from build123d import *

# Parameters (mm, degrees)
SKETCH1_R           = 10
BOSS_EXTRUDE1_DEPTH = 20
SKETCH2_R           = 24.856075314
SKETCH2_R_2         = 20
CUT_EXTRUDE3_DEPTH  = 20
SKETCH5_W           = 3
SKETCH5_H           = 20
CUT_EXTRUDE4_DEPTH  = 10
CUT_EXTRUDE5_START  = -20
SKETCH6_R           = 2.5
CUT_EXTRUDE5_DEPTH  = 25
SKETCH7_W           = 7
SKETCH7_H           = 8
CUT_EXTRUDE7_DEPTH  = 10
SKETCH8_R           = 0.5
CUT_EXTRUDE8_DEPTH  = 30
SKETCH9_W           = 2
SKETCH9_H           = 7.475145823
CUT_EXTRUDE9_DEPTH  = 23
SKETCH10_W          = 3
SKETCH10_H          = 24.206915905
CUT_EXTRUDE10_DEPTH = 2.5
SKETCH12_W          = 4
SKETCH12_H          = 4
CUT_EXTRUDE12_DEPTH = 15
BOSS_EXTRUDE7_DEPTH = 4
SKETCH39_R          = 2.5
CUT_EXTRUDE15_DEPTH = 12.5
BOSS_EXTRUDE8_DEPTH = 12.5
SKETCH42_R          = 0.6
CUT_EXTRUDE16_DEPTH = 33.5


with BuildPart() as part:
    # Sketch1 → Boss-Extrude1 (new body, symmetric)
    with BuildSketch(Plane(origin=(0, 0, 0), x_dir=(1, 0, 0), z_dir=(0, 1, 0))):
        Circle(SKETCH1_R)
    extrude(amount=BOSS_EXTRUDE1_DEPTH, both=True)

    # Sketch2 → Cut-Extrude3 (cut, symmetric)
    with BuildSketch(Plane.XY):
        Circle(SKETCH2_R)
        Circle(SKETCH2_R_2, mode=Mode.SUBTRACT)
    cut_extrude3 = extrude(amount=CUT_EXTRUDE3_DEPTH, both=True, mode=Mode.SUBTRACT)

    # Sketch5 → Cut-Extrude4 (cut)
    with BuildSketch(Plane(origin=(0, 20, 0), x_dir=(1, 0, 0), z_dir=(0, 1, 0))):
        Rectangle(SKETCH5_W, SKETCH5_H)
    cut_extrude4 = extrude(amount=-CUT_EXTRUDE4_DEPTH, mode=Mode.SUBTRACT)

    # Sketch6 → Cut-Extrude5 (cut)
    with BuildSketch(Plane.ZY.offset(-1.5).offset(CUT_EXTRUDE5_START)):
        with Locations((0, 13.943670675)):
            Circle(SKETCH6_R)
    cut_extrude5 = extrude(amount=CUT_EXTRUDE5_DEPTH, mode=Mode.SUBTRACT)

    # Sketch7 → Cut-Extrude7 (cut)
    with BuildSketch(Plane(origin=(0, 20, 0), x_dir=(1, 0, 0), z_dir=(0, 1, 0))):
        with Locations((5, 0)):
            Rectangle(SKETCH7_W, SKETCH7_H)
    cut_extrude7 = extrude(amount=-CUT_EXTRUDE7_DEPTH, mode=Mode.SUBTRACT)

    # Sketch8 → Cut-Extrude8 (cut)
    with BuildSketch(Plane(origin=(0, 10, 0), x_dir=(1, 0, 0), z_dir=(0, 1, 0))):
        with Locations((8, -3.414911062)):
            Circle(SKETCH8_R)
    cut_extrude8 = extrude(amount=-CUT_EXTRUDE8_DEPTH, mode=Mode.SUBTRACT)

    # Sketch9 → Cut-Extrude9 (cut)
    with BuildSketch(Plane(origin=(0, 10, 0), x_dir=(1, 0, 0), z_dir=(0, 1, 0))):
        with Locations((1.5, 7.737572912)):
            Rectangle(SKETCH9_W, SKETCH9_H)
    cut_extrude9 = extrude(amount=CUT_EXTRUDE9_DEPTH, mode=Mode.SUBTRACT)

    # Mirror2: Cut-Extrude3, Cut-Extrude4, Cut-Extrude5, Cut-Extrude7, Cut-Extrude8, Cut-Extrude9 across plane
    add(cut_extrude3.mirror(Plane.ZX), mode=Mode.SUBTRACT)
    add(cut_extrude4.mirror(Plane.ZX), mode=Mode.SUBTRACT)
    add(cut_extrude5.mirror(Plane.ZX), mode=Mode.SUBTRACT)
    add(cut_extrude7.mirror(Plane.ZX), mode=Mode.SUBTRACT)
    add(cut_extrude8.mirror(Plane.ZX), mode=Mode.SUBTRACT)
    add(cut_extrude9.mirror(Plane.ZX), mode=Mode.SUBTRACT)

    # Mirror3: Cut-Extrude8 across plane
    add(cut_extrude8.mirror(Plane.XY), mode=Mode.SUBTRACT)

    # Sketch10 → Cut-Extrude10 (cut)
    with BuildSketch(Plane(origin=(0, 10, 0), x_dir=(1, 0, 0), z_dir=(0, 1, 0))):
        with Locations((0, 0.041148578)):
            Rectangle(SKETCH10_W, SKETCH10_H)
    cut_extrude10 = extrude(amount=-CUT_EXTRUDE10_DEPTH, mode=Mode.SUBTRACT)

    # Mirror4: Cut-Extrude10 across plane
    add(cut_extrude10.mirror(Plane.ZX), mode=Mode.SUBTRACT)

    # Sketch12 → Cut-Extrude12 (cut, symmetric)
    with BuildSketch(Plane.XY):
        with Locations((-8, 0)):
            Rectangle(SKETCH12_W, SKETCH12_H)
        with Locations((8, 0)):
            Rectangle(SKETCH12_W, SKETCH12_H)
    extrude(amount=CUT_EXTRUDE12_DEPTH, both=True, mode=Mode.SUBTRACT)

    # Sketch37 → Boss-Extrude7 (add)
    with BuildSketch(Plane(origin=(0, 12.5, 0), x_dir=(1, 0, 0), z_dir=(0, 1, 0))):
        with BuildLine():
            Line((-2.5, 9.682458366), (-2.5, 12.247448714))
            ThreePointArc((-2.5, 12.247448714), (-7.90569415, -9.682458366), (12.5, 0))
            ThreePointArc((12.5, 0), (9.682458366, 7.90569415), (2.5, 12.247448714))
            Line((2.5, 12.247448714), (2.5, 9.682458366))
            ThreePointArc((2.5, 9.682458366), (7.90569415, 6.123724357), (10, 0))
            ThreePointArc((10, 0), (-6.123724357, -7.90569415), (-2.5, 9.682458366))
        make_face()
    boss_extrude7 = extrude(amount=-BOSS_EXTRUDE7_DEPTH)

    # Mirror5: Boss-Extrude7 across plane
    add(boss_extrude7.mirror(Plane.ZX))

    # Sketch39 → Cut-Extrude15 (cut)
    with BuildSketch(Plane(origin=(0, 0, 0), x_dir=(0, 0, -1), z_dir=(1, 0, 0))):
        with Locations((0, 13.943670675)):
            Circle(SKETCH39_R)
        with Locations((0, -13.943670675)):
            Circle(SKETCH39_R)
    extrude(amount=CUT_EXTRUDE15_DEPTH, mode=Mode.SUBTRACT)

    # Sketch41 → Boss-Extrude8 (add)
    with BuildSketch(Plane(origin=(0, 7.5, 0), x_dir=(1, 0, 0), z_dir=(0, 1, 0))):
        with BuildLine():
            Line((1.5, -6.25), (-1.5, -6.25))
            Line((-1.5, -6.25), (-1.5, -9.886859967))
            ThreePointArc((-1.5, -9.886859967), (0, -10), (1.5, -9.886859967))
            Line((1.5, -9.886859967), (1.5, -6.25))
        make_face()
    boss_extrude8 = extrude(amount=BOSS_EXTRUDE8_DEPTH)

    # Mirror6: Boss-Extrude8 across plane
    add(boss_extrude8.mirror(Plane.ZX))

    # Sketch42 → Cut-Extrude16 (cut, through all)
    with BuildSketch(Plane(origin=(0, 12.5, 0), x_dir=(1, 0, 0), z_dir=(0, 1, 0))):
        with Locations((11.25, 0)):
            Circle(SKETCH42_R)
    cut_extrude16 = extrude(amount=-CUT_EXTRUDE16_DEPTH, mode=Mode.SUBTRACT)

    # Mirror7: Cut-Extrude16 across plane
    add(cut_extrude16.mirror(Plane(origin=(0, 0, 0), x_dir=(0, 0, 1), z_dir=(1, 0, 0))), mode=Mode.SUBTRACT)


solid = part.part
Here's how the part is built. I have some questions about the finished solid (model axes, mm). A direction names the side the tool comes from. Round coordinates to 2 decimals unless told otherwise and drop trailing zeros. Loops run counter-clockwise (first coordinate to the right, second up) from the corner with the lowest first, then second, coordinate; pieces in that order, holes last. Notation, with made-up numbers: M 51.25,24.25 L 56.25,24.25 A30 cw 56.25,53.25 Z; hole C 81.5,-19 d9. An arc over 180 degrees is marked long. Write each question's results on one line, items separated by ' | '. Start each with the question number.
(1) I want a section at C-C (y = -9). Please give me the cut outline in (x, z), then the cut area to 3 significant figures.
(2) On a 3-axis mill with a long thin cutter (end or side, diameter ignored), from which of +Z, -Z, +X, -X, +Y, -Y can I reach the whole of each face in a straight line? I mean faces 1 (the cylindrical face through (10.084, 11.503, -0.542)), 2 (the flat face through (0.9, 8.5, 10.2)), 3 (the flat face through (0, -7.5, -2)), 4 (the flat face through (-8, 2, 0)). Say none if no direction works.
(3) I want a section at B-B (x = 0). Please give me the cut outline in (y, z).
(4) Thinking about a two-plate mould opening in X: for faces 5 (the cylindrical face through (-4.878, 19.396, -0.138)), 6 (the flat face through (5, -15, -4)), 7 (the flat face through (-7.5, 12.5, 7.4)), 8 (the cylindrical face through (8.74, 17.99, -0.03)), which applies, pulls with the +X half, pulls with the -X half, needs draft (parallel to the pull), parting line crosses it, or undercut?
(5) If I drill on probe 1 along Z at (x, y) = (8, 7.75); probe 2 along Y at (x, z) = (10.75, -4); probe 3 along X at (y, z) = (-9.5, -3.25), over which ranges is the centre line in solid material (lowest first)? Write a range as from..to.
(6) Will these pins go through, and if not, where does the flat tip stop? P1, Ø4, axis at x = 0.5, y = -1.5, coming from the +Z side; P2, Ø5, axis at y = -13, z = -0.5, coming from the +X side; P3, Ø8, axis at y = 13, z = 4.5, coming from the -X side; P4, Ø8, axis at x = -0.5, z = -9.5, coming from the +Y side.
(7) I want a section at D-D (x = -9). Please give me the cut outline in (y, z).
(8) I want a section at A-A (x = 9). Please give me the cut outline in (y, z), then the cut area to 3 significant figures.
Solved:
1) outline: M -2.5,-12.25 L -2.5,-9.68 A10 ccw -1.5,-9.89 L -1.5,6.25 L 1.5,6.25 L 1.5,-9.89 A10 ccw 2.5,-9.68 L 2.5,-12.25 A12.5 ccw long Z; hole C -11.25,0 d1.2; hole C 8,-3.41 d1; hole C 8,3.41 d1; hole C 11.25,0 d1.2 | area: 426 mm²
2) face 1: +X | face 2: none | face 3: -Z, -Y | face 4: +Z, -Z, -X
3) outline: M -20,6.25 L -7.5,6.25 L -7.5,-10 L 7.5,-10 L 7.5,6.25 L 20,6.25 L 20,10 L 12.5,10 L 12.5,12.5 L 8.5,12.5 L 8.5,10 L -8.5,10 L -8.5,12.5 L -12.5,12.5 L -12.5,10 L -20,10 Z
4) face 5: pulls with the -X half | face 6: undercut | face 7: needs draft | face 8: pulls with the +X half
5) probe 1: z = -6..-3.91, -2.91..2.91, 3.91..6 | probe 2: y = -12.5..-8.5, 8.5..12.5 | probe 3: x = -12.07..-1.5, 1.5..7.53, 8.47..12.07
6) P1: stops at z = 10 | P2: stops at x = 12.5 | P3: stops at x = -12.49 | P4: stops at y = 19.94
7) outline: M -17.86,-4.36 L -12.5,-4.36 L -12.5,-8.67 L -8.5,-8.67 L -8.5,-4.36 L -2,-4.36 L -2,4.36 L -8.5,4.36 L -8.5,8.67 L -12.5,8.67 L -12.5,4.36 L -17.86,4.36 Z; M 2,-4.36 L 8.5,-4.36 L 8.5,-8.67 L 12.5,-8.67 L 12.5,-4.36 L 17.86,-4.36 L 17.86,4.36 L 12.5,4.36 L 12.5,8.67 L 8.5,8.67 L 8.5,4.36 L 2,4.36 Z
8) outline: M -17.86,-4.36 L -12.5,-4.36 L -12.5,-8.67 L -8.5,-8.67 L -8.5,-4.36 L -2,-4.36 L -2,4.36 L -8.5,4.36 L -8.5,8.67 L -12.5,8.67 L -12.5,4.36 L -17.86,4.36 Z; M 2,-4.36 L 8.5,-4.36 L 8.5,-8.67 L 12.5,-8.67 L 12.5,-4.36 L 17.86,-4.36 L 17.86,4.36 L 12.5,4.36 L 12.5,8.67 L 8.5,8.67 L 8.5,4.36 L 2,4.36 Z; hole C -13.94,0 d5; hole C 13.94,0 d5 | area: 306 mm²
